```python
from build123d import *

# Parameters (mm, degrees)
SKETCH1_R          = 3.4036
EXTRUDE1_DEPTH     = 76.2
CUT_EXTRUDE1_DEPTH = 88.016609357
CUT_EXTRUDE2_DEPTH = 88.016609357
CUT_EXTRUDE3_REACH = 89.017
CUT_EXTRUDE5_DEPTH = 88.016609357


with BuildPart() as part:
    # Sketch1 → Extrude1 (new, symmetric)
    with BuildSketch(Plane.XY):
        with BuildLine():
            Line((-20, 16.952), (-20, 4.7625))
            ThreePointArc((-20, 4.7625), (-19.776815367, 4.223684633), (-19.238, 4.0005))
            Line((-19.238, 4.0005), (-16.2662, 4.0005))
            ThreePointArc((-16.2662, 4.0005), (-15.727384633, 4.223684633), (-15.5042, 4.7625))
            Line((-15.5042, 4.7625), (-15.5042, 10.485558599))
            ThreePointArc((-15.5042, 10.485558599), (-15.033804775, 11.189554802), (-14.203384633, 11.024373966))
            Line((-14.203384633, 11.024373966), (-8.635059555, 5.456048889))
            ThreePointArc((-8.635059555, 5.456048889), (-7.985348265, 4.483687227), (-7.7572, 3.336708444))
            Line((-7.7572, 3.336708444), (-7.7572, -3.336708444))
            ThreePointArc((-7.7572, -3.336708444), (-7.985348265, -4.483687227), (-8.635059555, -5.456048889))
            Line((-8.635059555, -5.456048889), (-14.203384633, -11.024373966))
            ThreePointArc((-14.203384633, -11.024373966), (-15.033804775, -11.189554802), (-15.5042, -10.485558599))
            Line((-15.5042, -10.485558599), (-15.5042, -4.7625))
            ThreePointArc((-15.5042, -4.7625), (-15.727384633, -4.223684633), (-16.2662, -4.0005))
            Line((-16.2662, -4.0005), (-19.238, -4.0005))
            ThreePointArc((-19.238, -4.0005), (-19.776815367, -4.223684633), (-20, -4.7625))
            Line((-20, -4.7625), (-20, -16.952))
            ThreePointArc((-20, -16.952), (-19.107261469, -19.107261469), (-16.952, -20))
            Line((-16.952, -20), (-4.7625, -20))
            ThreePointArc((-4.7625, -20), (-4.223684633, -19.776815367), (-4.0005, -19.238))
            Line((-4.0005, -19.238), (-4.0005, -16.2662))
            ThreePointArc((-4.0005, -16.2662), (-4.223684633, -15.727384633), (-4.7625, -15.5042))
            Line((-4.7625, -15.5042), (-10.485558599, -15.5042))
            ThreePointArc((-10.485558599, -15.5042), (-11.189554802, -15.033804775), (-11.024373966, -14.203384633))
            Line((-11.024373966, -14.203384633), (-5.456048889, -8.635059555))
            ThreePointArc((-5.456048889, -8.635059555), (-4.483687227, -7.985348265), (-3.336708444, -7.7572))
            Line((-3.336708444, -7.7572), (3.336708444, -7.7572))
            ThreePointArc((3.336708444, -7.7572), (4.483687227, -7.985348265), (5.456048889, -8.635059555))
            Line((5.456048889, -8.635059555), (11.024373966, -14.203384633))
            ThreePointArc((11.024373966, -14.203384633), (11.189554802, -15.033804775), (10.485558599, -15.5042))
            Line((10.485558599, -15.5042), (4.7625, -15.5042))
            ThreePointArc((4.7625, -15.5042), (4.223684633, -15.727384633), (4.0005, -16.2662))
            Line((4.0005, -16.2662), (4.0005, -19.238))
            ThreePointArc((4.0005, -19.238), (4.223684633, -19.776815367), (4.7625, -20))
            Line((4.7625, -20), (16.952, -20))
            ThreePointArc((16.952, -20), (19.107261469, -19.107261469), (20, -16.952))
            Line((20, -16.952), (20, -4.7625))
            ThreePointArc((20, -4.7625), (19.776815367, -4.223684633), (19.238, -4.0005))
            Line((19.238, -4.0005), (16.2662, -4.0005))
            ThreePointArc((16.2662, -4.0005), (15.727384633, -4.223684633), (15.5042, -4.7625))
            Line((15.5042, -4.7625), (15.5042, -10.485558599))
            ThreePointArc((15.5042, -10.485558599), (15.033804775, -11.189554802), (14.203384633, -11.024373966))
            Line((14.203384633, -11.024373966), (8.635059555, -5.456048889))
            ThreePointArc((8.635059555, -5.456048889), (7.985348265, -4.483687227), (7.7572, -3.336708444))
            Line((7.7572, -3.336708444), (7.7572, 3.336708444))
            ThreePointArc((7.7572, 3.336708444), (7.985348265, 4.483687227), (8.635059555, 5.456048889))
            Line((8.635059555, 5.456048889), (14.203384633, 11.024373966))
            ThreePointArc((14.203384633, 11.024373966), (15.033804775, 11.189554802), (15.5042, 10.485558599))
            Line((15.5042, 10.485558599), (15.5042, 4.7625))
            ThreePointArc((15.5042, 4.7625), (15.727384633, 4.223684633), (16.2662, 4.0005))
            Line((16.2662, 4.0005), (19.238, 4.0005))
            ThreePointArc((19.238, 4.0005), (19.776815367, 4.223684633), (20, 4.7625))
            Line((20, 4.7625), (20, 16.952))
            ThreePointArc((20, 16.952), (19.107261469, 19.107261469), (16.952, 20))
            Line((16.952, 20), (4.7625, 20))
            ThreePointArc((4.7625, 20), (4.223684633, 19.776815367), (4.0005, 19.238))
            Line((4.0005, 19.238), (4.0005, 16.2662))
            ThreePointArc((4.0005, 16.2662), (4.223684633, 15.727384633), (4.7625, 15.5042))
            Line((4.7625, 15.5042), (10.485558599, 15.5042))
            ThreePointArc((10.485558599, 15.5042), (11.189554802, 15.033804775), (11.024373966, 14.203384633))
            Line((11.024373966, 14.203384633), (5.456048889, 8.635059555))
            ThreePointArc((5.456048889, 8.635059555), (4.483687227, 7.985348265), (3.336708444, 7.7572))
            Line((3.336708444, 7.7572), (-3.336708444, 7.7572))
            ThreePointArc((-3.336708444, 7.7572), (-4.483687227, 7.985348265), (-5.456048889, 8.635059555))
            Line((-5.456048889, 8.635059555), (-11.024373966, 14.203384633))
            ThreePointArc((-11.024373966, 14.203384633), (-11.189554802, 15.033804775), (-10.485558599, 15.5042))
            Line((-10.485558599, 15.5042), (-4.7625, 15.5042))
            ThreePointArc((-4.7625, 15.5042), (-4.223684633, 15.727384633), (-4.0005, 16.2662))
            Line((-4.0005, 16.2662), (-4.0005, 19.238))
            ThreePointArc((-4.0005, 19.238), (-4.223684633, 19.776815367), (-4.7625, 20))
            Line((-4.7625, 20), (-16.952, 20))
            ThreePointArc((-16.952, 20), (-19.107261469, 19.107261469), (-20, 16.952))
        make_face()
        with Locations(Location((0, 0, 0), (0, 0, 180))):
            Circle(SKETCH1_R, mode=Mode.SUBTRACT)
    extrude(amount=EXTRUDE1_DEPTH, both=True)

    # Sketch3 → Cut-Extrude1 (cut, through all)
    with BuildSketch(Plane(origin=(0, 16.952, 0), x_dir=(1, 0, 0), z_dir=(0, 1, 0))):
        Polygon((20, -76.2), (-20, -36.2), (-20, -76.2), align=None)
    extrude(amount=-CUT_EXTRUDE1_DEPTH, mode=Mode.SUBTRACT)

    # Sketch4 → Cut-Extrude2 (cut, through all)
    with BuildSketch(Plane(origin=(0, 16.952, 0), x_dir=(-1, 0, 0), z_dir=(0, -1, 0))):
        Polygon((20, -36.2), (-20, -76.2), (20, -76.2), align=None)
    extrude(amount=-CUT_EXTRUDE2_DEPTH, mode=Mode.SUBTRACT)

    # Sketch5 → Cut-Extrude3 (cut, up to next)
    with BuildSketch(Plane(origin=(0, 16.952, 0), x_dir=(1, 0, 0), z_dir=(0, 1, 0)), mode=Mode.PRIVATE) as cut_extrude3_sk1:
        Polygon((20, 76.2), (-20, 76.2), (-20, 36.2), align=None)
    cut_extrude3_tool1 = extrude(cut_extrude3_sk1.sketch, amount=-CUT_EXTRUDE3_REACH, mode=Mode.PRIVATE) & part.part
    add(cut_extrude3_tool1.solids().sort_by_distance((-6.666667, 16.952, -62.866667))[0], mode=Mode.SUBTRACT)

    # Sketch7 → Cut-Extrude5 (cut, through all)
    with BuildSketch(Plane(origin=(0, 16.952, 0), x_dir=(-1, 0, 0), z_dir=(0, -1, 0))):
        Polygon((20, 36.2), (20, 76.2), (-20, 76.2), align=None)
    extrude(amount=-CUT_EXTRUDE5_DEPTH, mode=Mode.SUBTRACT)


solid = part.part
```
The model under review builds one solid part; all positions refer to its coordinate system, in mm. A direction names the side the tool comes from. Round coordinates to 2 decimals unless told otherwise and drop trailing zeros. Loops run counter-clockwise (first coordinate to the right, second up) from the corner with the lowest first, then second, coordinate; pieces in that order, holes last. Notation, with made-up numbers: M 42,29.25 L 55,29.25 A23 ccw 55,50.25 Z; hole C -30,-26.5 d4. An arc over 180 degrees is marked long. Put each result on its own line as item: value.
Q1. To check wall thickness, follow L1, parallel to X at y = 8, z = -46; L2, parallel to Y at x = 0, z = 35; L3, parallel to Y at x = -7, z = -2.5. State the ranges of each line that lie inside material, in increasing order.
Result set:
L1: x = -10.2 to -4.52, 4.52 to 11.18, 15.5 to 20
L2: y = -7.76 to -3.4, 3.4 to 7.76
L3: y = -20 to -15.5, -10.18 to 10.18, 15.5 to 20
Q2. Consider section B-B, the plane y = 0. Give the boundary of the cut face in (x, z), then the cut area to 3 significant figures.
Result set:
outline: M -7.76,-48.44 L -3.4,-52.8 L -3.4,52.8 L -7.76,48.44 Z; M 3.4,-59.6 L 7.76,-63.96 L 7.76,63.96 L 3.4,59.6 Z
area: 979 mm²
Q3. Consider section A-A, the plane x = 0. Give the boundary of the cut face in (y, z), then the cut area to 3 significant figures.
Result set:
outline: M -7.76,-56.2 L -3.4,-56.2 L -3.4,56.2 L -7.76,56.2 Z; M 3.4,-56.2 L 7.76,-56.2 L 7.76,56.2 L 3.4,56.2 Z
area: 979 mm²
Q4. Mouldability with a two-part tool opening along Y and no side actions: class faces 5 (the flat face through (0, 7.757, 1)), 6 (the flat face through (11.38, 8.2, 0.99)), 7 (the flat face through (7.757, 0, 1)), 8 (the flat face through (4, -18, 1)) as released by +Y, released by -Y, zero draft, split by the parting line, or undercut.
Result set:
face 5: released by +Y
face 6: undercut
face 7: undercut
face 8: zero draft
Q5. For pin 1 (2.5 mm diameter, centred on y = 18.5, z = -13.5, fed in from +X); pin 2 (5.5 mm diameter, centred on y = 1, z = -8.5, fed in from -X); pin 3 (8 mm diameter, centred on x = 13, y = 8, fed in from +Z), all flat-tipped, find the tip position at first contact; note any pin that passes through.
Result set:
pin 1: stops at x = 19.99
pin 2: stops at x = -7.79
pin 3: stops at z = 73.2
Q6. Machinability: for faces 1 (the flat face through (18, -4, 1)), 2 (the flat face through (-18, -4, 1)), 3 (the flat face through (-4, -18, 1)), 4 (the flat face through (-15.504, 8, 1)), which of the approach directions +Z, -Z, +X, -X, +Y, -Y give a long, thin tool a straight path to every point of the face, cutting with its end or side? Answer none if there is none.
Result set:
face 1: +Z, -Z, +X
face 2: +Z, -Z, -X
face 3: +Z, -Z, -Y
face 4: +Z, -Z
